Input: part model. Units: mm. Frame: model coordinates. Coordinates: 2 decimals unless noted, no trailing zeros. Loops run counter-clockwise (first coordinate to the right, second up) from the corner with the lowest first, then second, coordinate; pieces in that order, holes last. Notation, with made-up numbers: M 53,-20.5 L 104,-20.5 A11 cw 104,-10.5 Z; hole C 56.5,-37 d7. An arc over 180 degrees is marked long. Use a Markdown table: item, result. Add a question column.
1. Line query: L1, parallel to Z at x = 25, y = -3.9; L2, parallel to X at y = -0.8, z = 274. Output: solid intervals per line, ascending. Write a range as [from, to].
2. Section B-B on y = -3.15. Output: boundary loops of the cut face in (x, z).
3. Section A-A on x = 25.4. Output: boundary loops of the cut face in (y, z), then the cut area to 3 significant figures.
```python
from build123d import *

# Parameters (mm, degrees)
F0_W     = 50.8
F0_H     = 292.1
F1_DEPTH = 4.7625


with BuildPart() as f1:
    # F0 (on Front) → F1 (new body)
    with BuildSketch(Plane.XZ):
        with Locations((25.4, 146.05)):
            Rectangle(F0_W, F0_H)
        with BuildLine():
            ThreePointArc((29.718, 15.08125), (25.4, 10.76325), (21.082, 15.08125))
            Line((21.082, 15.08125), (21.082, 23.01875))
            ThreePointArc((21.082, 23.01875), (25.4, 27.33675), (29.718, 23.01875))
            Line((29.718, 23.01875), (29.718, 15.08125))
        make_face(mode=Mode.SUBTRACT)
        with BuildLine():
            ThreePointArc((29.718, 269.08125), (25.4, 264.76325), (21.082, 269.08125))
            Line((21.082, 269.08125), (21.082, 277.01875))
            ThreePointArc((21.082, 277.01875), (25.4, 281.33675), (29.718, 277.01875))
            Line((29.718, 277.01875), (29.718, 269.08125))
        make_face(mode=Mode.SUBTRACT)
    extrude(amount=F1_DEPTH)


solid = f1.part
```
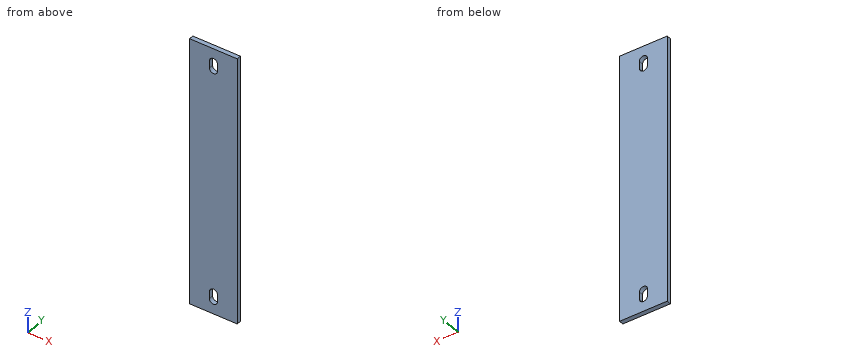
Answers below:
| question | item | result |
|---|---|---|
| 1 | L1 | z = [0, 10.78], [27.32, 264.78], [281.32, 292.1] |
| 1 | L2 | x = [0, 21.08], [29.72, 50.8] |
| 2 | outline | M 0,0 L 50.8,0 L 50.8,292.1 L 0,292.1 Z; hole M 21.08,15.08 A4.32 ccw 29.72,15.08 L 29.72,23.02 A4.32 ccw 21.08,23.02 Z; hole M 21.08,269.08 A4.32 ccw 29.72,269.08 L 29.72,277.02 A4.32 ccw 21.08,277.02 Z |
| 3 | outline | M -4.76,0 L 0,0 L 0,10.76 L -4.76,10.76 Z; M -4.76,27.34 L 0,27.34 L 0,264.76 L -4.76,264.76 Z; M -4.76,281.34 L 0,281.34 L 0,292.1 L -4.76,292.1 Z |
| 3 | area | 1,230 mm² |
